Part model, mm, in its own coordinate system. A direction names the side the tool comes from. Round coordinates to 2 decimals unless told otherwise and drop trailing zeros. Order: outer loops, then holes, each group sorted by start corner. A loop starts at its lowest first (then second) coordinate and runs counter-clockwise, first axis right, second up. Notation, with made-up numbers: (84.25, 37) - (128.25, 37) arc R23 ccw to (128.25, 56) - close; hole circle Ø6 at (87, -30.5). An arc over 180 degrees is marked (long way). Answer as a JSON object with one key per item and string values.
Autodesk Inventor part; units mm, degrees
ref_plane "YZ Plane" through (0, 0, 0) normal (1, 0, 0) x (0, 1, 0)
ref_plane "XZ Plane" through (0, 0, 0) normal (0, 1, 0) x (-1, 0, 0)
ref_plane "XY Plane" through (0, 0, 0) normal (0, 0, 1) x (1, 0, 0)
sketch "Boceto1" plane through (0, 0, 0) normal (0, 0, 1) x (1, 0, 0)
  line L0 (0, 0) -> (0, 49.6834)
  line L1 (0.0978, 50.3011) -> (13.4493, 91.4177)
  line L2 (58.8982, 92.8) -> (58.8982, 0)
  arc A0 (15.3516, 92.8) -> (13.4493, 91.4177) centre (15.3516, 90.8) ccw
  arc A1 (0.0978, 50.3011) -> (0, 49.6834) centre (2, 49.6834) ccw
  line L3 (2.9528, 52.6177) -> (13.9285, 86.4177)
  line L4 (15.8307, 87.8) -> (54.8982, 87.8)
  line L5 (56.8982, 85.8) -> (56.8982, 52)
  line L6 (54.8982, 50) -> (4.8551, 50)
  arc A2 (15.8307, 87.8) -> (13.9285, 86.4177) centre (15.8307, 85.8) ccw
  arc A3 (56.8982, 85.8) -> (54.8982, 87.8) centre (54.8982, 85.8) ccw
  arc A4 (54.8982, 50) -> (56.8982, 52) centre (54.8982, 52) ccw
  arc A5 (2.9528, 52.6177) -> (4.8551, 50) centre (4.8551, 52) ccw
  line L7 (0, 0) -> (58.8982, 0)
  line L8 (15.3516, 92.8) -> (58.8982, 92.8)
  point P0 (0, 50)
  point P1 (13.8982, 92.8)
  point P2 (2.1028, 50)
  point P3 (0.0246, 49.9961)
  dimension "d31" = 45
  dimension "d32" = 50
  dimension "d33" = 45
  dimension "d43" = 2
  dimension "d48" = 2
  dimension "d49" = 2
  dimension "d50" = 2
  dimension "d57" = 92.8
  dimension "d58" = 5
  dimension "d59" = 13.4493
  dimension "d60" = 162.01
extrude "Extrusión3" add sketch "Boceto1" against normal blind 8
sketch "Boceto2" plane through (58.8982, 0, 0) normal (1, 0, 0) x (0, 0, -1)
  circle A0 centre (4, 10) radius 1.5
  circle A1 centre (4, 89.8) radius 1.5
  line L0 (0, 0) -> (8, 0)
  line L1 (0, 0) -> (0, 49.6834)
  line L2 (0, 92.8) -> (8, 92.8)
  line L3 (0, 92.8) -> (0, 0)
  dimension "d61" = 3
  dimension "d62" = 10
  dimension "d63" = 4
  dimension "d64" = 3
  dimension "d65" = 4
extrude "Extrusión4" add sketch "Boceto2" along normal blind 10
sketch "Boceto3" plane through (0, 0, -8) normal (0, 0, -1) x (-1, 0, 0)
  circle A0 centre (-29.4582, 10) radius 4
  line L0 (-58.8982, 0) -> (0, 0)
  line L1 (-58.8982, 92.8) -> (-58.8982, 0)
  dimension "d68" = 10
  dimension "d69" = 29.44
  dimension "d72" = 8
extrude "Extrusión5" add sketch "Boceto3" along normal blind 10
properties part number "Puerta"
Item 1: Tool access for faces 5 (the flat face through (56.898, 69, -4)), 6 (the flat face through (68.898, 10, -4)), 7 (the cylindrical face through (63.83, 91.13, -4.69)): list every direction of +Z, -Z, +X, -X, +Y, -Y with a clear straight run to the whole face (end or side of a thin tool).
Taken from the geometry:
{"face 5": "+Z, -Z", "face 6": "+Z, -Z, +X, +Y, -Y", "face 7": "+X"}
Item 2: Probe L1, parallel to Y at x = 34.5, z = -4.25; L2, parallel to Z at x = 58, y = 50.5; L3, parallel to X at y = 28, z = -2.5. List the from-to ranges inside material, lowest first. Write a range as from..to.
Taken from the geometry:
{"L1": "0..50, 87.8..92.8", "L2": "-8..0", "L3": "0..58.9"}
Item 3: Cut at C-C (z = -9.75). Write the cut outline in (x, y), plus the area to 3 significant figures.
Taken from the geometry:
{"outline": "circle Ø8 at (29.46, 10)", "area": "50.3 mm2"}
Item 4: Drop flat-ended pins along their axis: P1, Ø3, axis at x = 60.5, z = -6.5, coming from the -Y side; P2, Ø6.5, axis at y = 61.5, z = -3.5, coming from the -X side; P3, Ø3, axis at y = 16, z = -12, coming from the -X side; P4, Ø9, axis at y = 46.5, z = -4.5, coming from the +X side. Give the stop position or say it passes through.
Taken from the geometry:
{"P1": "y = 8.88", "P2": "x = 2.68", "P3": "through", "P4": "x = 58.9"}
Item 5: Two-plate mould, pull along X, no slides. Class faces 1 (the cylindrical face through (33.454, 9.824, -12.93)), 2 (the cylindrical face through (14.67, 87.43, -3.94)), 3 (the cylindrical face through (3.22, 50.85, -3.94)), 4 (the flat face through (0, 24, -4)): pulls with the +X half, pulls with the -X half, needs draft (parallel to the pull), parting line crosses it, or undercut.
Taken from the geometry:
{"face 1": "parting line crosses it", "face 2": "undercut", "face 3": "undercut", "face 4": "pulls with the -X half"}
Item 6: Cut at B-B (y = 10). Write the cut outline in (x, z), plus the area to 3 significant figures.
Taken from the geometry:
{"outline": "(0, -8) - (25.46, -8) - (25.46, -18) - (33.46, -18) - (33.46, -8) - (58.9, -8) - (58.9, -5.5) - (68.9, -5.5) - (68.9, -2.5) - (58.9, -2.5) - (58.9, 0) - (0, 0) - close", "area": "581 mm2"}
Item 7: Cut at D-D (y = 63.5). Write the cut outline in (x, z).
Taken from the geometry:
{"outline": "(4.38, -8) - (6.49, -8) - (6.49, 0) - (4.38, 0) - close; (56.9, -8) - (58.9, -8) - (58.9, 0) - (56.9, 0) - close"}
Item 8: Cut at A-A (x = 47.5). Write the cut outline in (y, z), plus the area to 3 significant figures.
Taken from the geometry:
{"outline": "(0, -8) - (50, -8) - (50, 0) - (0, 0) - close; (87.8, -8) - (92.8, -8) - (92.8, 0) - (87.8, 0) - close", "area": "440 mm2"}
